Could you check a few things on this model? Use its own coordinates, in mm. Face numbers are marked on the shaded views. A direction names the side the tool comes from. Give positions to 0.01 mm unless a question says otherwise; leave off trailing zeros. Write each loop counter-clockwise with the first axis right and the second up, starting at its lowest first coordinate (ties: lowest second). Pieces come first, ordered by that corner, then holes. Notation, with made-up numbers: M 67.25,78 L 92.25,78 A22 cw 92.25,84 Z; hole C 82,48.25 d7. An arc over 180 degrees is marked long. Answer as a JSON object with one key per item and string values. Group by question number.
```python
from build123d import *

# Parameters (mm, degrees)
SKETCH1_R               = 2.500000508
BOSS_EXTRUDE1_DEPTH     = 12
SKETCH2_R               = 10
BOSS_EXTRUDE2_DEPTH     = 8
CUT_EXTRUDE5_DEPTH      = 6.8
SKETCH10_R              = 2.500000508
CUT_EXTRUDE6_DEPTH      = 10
CHAMFER1_SIZE           = 1
SKETCH11_R              = 1.7
CUT_EXTRUDE7_DEPTH      = 10
CUT_EXTRUDE7_DEPTH_BACK = 2


with BuildPart() as part:
    # Sketch1 → Boss-Extrude1 (new body)
    with BuildSketch(Plane.XY.offset(15)):
        Polygon((-0.020282, 4.479718), (1.693392048, 4.157458362), (2.715058109, 5.335905553), (3.851065458, 4.576848343), (3.153297436, 3.181980515), (4.137176, 1.742358), (5.692891, 1.853219), (5.959435, 0.513206), (4.479718, 0.020282), (4.157458362, -1.693392048), (5.335905553, -2.715058109), (4.576848343, -3.851065458), (3.181980515, -3.153297436), (1.742358, -4.137176), (1.853219, -5.692891), (0.513206, -5.959435), (0.020282, -4.479718), (-1.693392048, -4.157458362), (-2.715058109, -5.335905553), (-3.851065458, -4.576848343), (-3.153297436, -3.181980515), (-4.137176, -1.742358), (-5.692891, -1.853219), (-5.959435, -0.513206), (-4.479718, -0.020282), (-4.157458362, 1.693392048), (-5.335905553, 2.715058109), (-4.576848343, 3.851065458), (-3.181980515, 3.153297436), (-1.742358, 4.137176), (-1.853219, 5.692891), (-0.513206, 5.959435), align=None)
        Circle(SKETCH1_R, mode=Mode.SUBTRACT)
    extrude(amount=-BOSS_EXTRUDE1_DEPTH)

    # Sketch2 → Boss-Extrude2 (add)
    with BuildSketch(Plane(origin=(0, 0, 3), x_dir=(-1, 0, 0), z_dir=(0, 0, -1))):
        Circle(SKETCH2_R)
    extrude(amount=BOSS_EXTRUDE2_DEPTH)

    # Sketch9 → Cut-Extrude5 (cut)
    with BuildSketch(Plane(origin=(0, 0, -5), x_dir=(-1, 0, 0), z_dir=(0, 0, -1))):
        Polygon((3.802129012, 2.564951973), (4.58587219, 5.460767338), (-1.20575854, 7.028253696), (-1.989501719, 4.13243833), align=None)
    extrude(amount=-CUT_EXTRUDE5_DEPTH, mode=Mode.SUBTRACT)

    # Sketch10 → Cut-Extrude6 (cut)
    with BuildSketch(Plane.XY.offset(3)):
        Circle(SKETCH10_R)
    extrude(amount=-CUT_EXTRUDE6_DEPTH, mode=Mode.SUBTRACT)

    # Chamfer1
    chamfer1_edges = [part.edges().sort_by_distance(p)[0] for p in [
        (10, 0, 3),
    ]]
    chamfer(chamfer1_edges, length=CHAMFER1_SIZE)

    # Sketch11 → Cut-Extrude7 (cut, two sides)
    with BuildSketch(Plane(origin=(-0.906313646, 3.348695152, 0), x_dir=(0.965271788, 0.261247726, 0), z_dir=(-0.261247726, 0.965271788, 0))) as cut_extrude7_sk:
        with Locations((0, 1.6)):
            Circle(SKETCH11_R)
    extrude(amount=CUT_EXTRUDE7_DEPTH, mode=Mode.SUBTRACT)
    extrude(cut_extrude7_sk.sketch, amount=-CUT_EXTRUDE7_DEPTH_BACK, mode=Mode.SUBTRACT)


solid = part.part
```
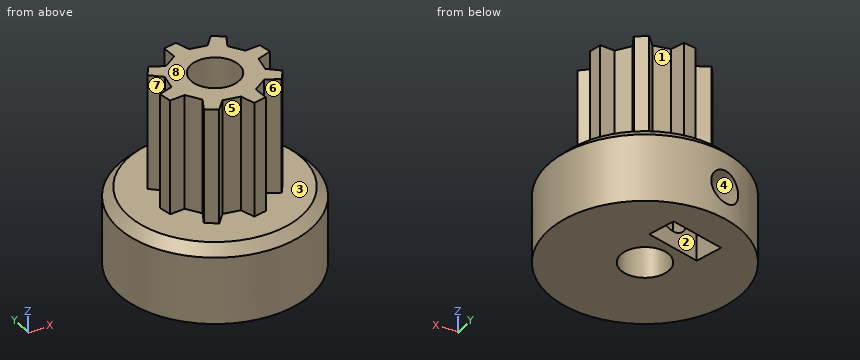
1) Please list where these lines run through material, in increasing order: line 1 along Y through (x, z) = (0, 9.5); line 2 along Z through (x, y) = (4.75, 0); line 3 along Y through (x, z) = (0, 0). Write a range as from..to.
2) If we section it at B-B, the plane z = 0.75: List the corners of the cut face in (x, y) for me, plus the area to 3 significant figures.
3) If we section it at C-C, the plane z = -3: List the corners of the cut face in (x, y) for me, plus the area to 3 significant figures.
4) For the marked faces 1, 2, 3, 4 and 5, which set-ups out of +Z, -Z, +X, -X, +Y, -Y let a thin tool reach every point of the face, with its end or its side?
5) We'd pull the mould along X, two halves only. Please class the marked faces 6, 7 and 8: released by +X, released by -X, zero draft, split by the parting line, or undercut.
6) I'm going to push flat-ended pins straight in: pin 1 (6 mm diameter, centred on y = -3, z = 8, fed in from +X); pin 2 (3 mm diameter, centred on x = 0, y = 0, fed in from +Z); pin 3 (6 mm diameter, centred on y = 6, z = 0.5, fed in from +X); pin 4 (5 mm diameter, centred on y = -3, z = 10, fed in from -X). Where does each tip first touch, or does it pass through?
Taken from the geometry:
{
 "1": {"line 1": "-4.48..-2.5, 2.5..4.48", "line 2": "-5..3", "line 3": "-10..-2.5, 2.5..3.59, 6.7..10"},
 "2": {"outline": "C 0,0 d20; hole M -4.59,5.46 L -3.8,2.56 L 1.99,4.13 L 1.21,7.03 Z; hole C 0,0 d5", "area": "277 mm²"},
 "3": {"outline": "M -4.59,5.46 L -2.62,5.99 L -3.53,9.36 A10 ccw long -1.67,9.86 L -0.76,6.5 L 1.21,7.03 L 1.99,4.13 L 0.02,3.6 L 0.33,2.48 A2.5 cw long -1.53,1.97 L -1.84,3.1 L -3.8,2.56 Z", "area": "268 mm²"},
 "4": {"face 1": "+Z, +Y", "face 2": "-Z", "face 3": "+Z", "face 4": "none", "face 5": "+Z, -Y"},
 "5": {"face 6": "undercut", "face 7": "released by -X", "face 8": "zero draft"},
 "6": {"pin 1": "x = 5.34", "pin 2": "through", "pin 3": "x = 9.54", "pin 4": "x = -5.96"}
}
